```python
from build123d import *

# Parameters (mm, degrees)
SKETCH1_R           = 0.46989906
SKETCH1_R_2         = 0.2499995
BOSS_EXTRUDE1_DEPTH = 1.6764


with BuildPart() as part:
    # Sketch1 → Boss-Extrude1 (new body)
    with BuildSketch(Plane(origin=(0, 0, 0), x_dir=(1, 0, 0), z_dir=(0, 1, 0))):
        with BuildLine():
            Line((73.134188992, 51.586783601), (72.472390316, 51.586783601))
            ThreePointArc((72.472390316, 51.586783601), (72.466796066, 51.573277888), (72.453290354, 51.567683639))
            ThreePointArc((72.453290354, 51.567683639), (72.439692672, 51.573370488), (72.434192176, 51.587044615))
            ThreePointArc((72.434192176, 51.587044615), (71.958321344, 51.791813191), (71.753552768, 52.267684022))
            ThreePointArc((71.753552768, 52.267684022), (71.739878641, 52.273184519), (71.734191792, 52.286782201))
            ThreePointArc((71.734191792, 52.286782201), (71.739786041, 52.300287913), (71.753291754, 52.305882163))
            Line((71.753291754, 52.305882163), (71.753291754, 53.067680639))
            ThreePointArc((71.753291754, 53.067680639), (71.739786041, 53.073274888), (71.734191792, 53.086780601))
            ThreePointArc((71.734191792, 53.086780601), (71.73975368, 53.100253874), (71.753200111, 53.105880343))
            ThreePointArc((71.753200111, 53.105880343), (71.167492925, 54.500977772), (69.772395496, 55.086684958))
            ThreePointArc((69.772395496, 55.086684958), (69.766769027, 55.073238527), (69.753295754, 55.067676639))
            ThreePointArc((69.753295754, 55.067676639), (69.739790041, 55.073270888), (69.734195792, 55.086776601))
            Line((69.734195792, 55.086776601), (57.253320754, 55.086776601))
            ThreePointArc((57.253320754, 55.086776601), (55.845892561, 54.507714506), (55.253416396, 53.105880343))
            ThreePointArc((55.253416396, 53.105880343), (55.266862828, 53.100253874), (55.272424716, 53.086780601))
            ThreePointArc((55.272424716, 53.086780601), (55.266830466, 53.073274888), (55.253324754, 53.067680639))
            Line((55.253324754, 53.067680639), (55.253324754, 41.105904563))
            ThreePointArc((55.253324754, 41.105904563), (55.266830466, 41.100310313), (55.272424716, 41.086804601))
            ThreePointArc((55.272424716, 41.086804601), (55.266862828, 41.073331328), (55.253416396, 41.067704859))
            ThreePointArc((55.253416396, 41.067704859), (55.845892561, 39.665870695), (57.253320754, 39.086808601))
            Line((57.253320754, 39.086808601), (69.734195792, 39.086808601))
            ThreePointArc((69.734195792, 39.086808601), (69.739790041, 39.100314313), (69.753295754, 39.105908563))
            ThreePointArc((69.753295754, 39.105908563), (69.766769027, 39.100346675), (69.772395496, 39.086900243))
            ThreePointArc((69.772395496, 39.086900243), (71.167492925, 39.672607429), (71.753200111, 41.067704859))
            ThreePointArc((71.753200111, 41.067704859), (71.73975368, 41.073331328), (71.734191792, 41.086804601))
            ThreePointArc((71.734191792, 41.086804601), (71.739786041, 41.100310313), (71.753291754, 41.105904563))
            Line((71.753291754, 41.105904563), (71.753291754, 41.867703039))
            ThreePointArc((71.753291754, 41.867703039), (71.739786041, 41.873297288), (71.734191792, 41.886803001))
            ThreePointArc((71.734191792, 41.886803001), (71.739878641, 41.900400683), (71.753552768, 41.905901179))
            ThreePointArc((71.753552768, 41.905901179), (71.958321344, 42.381772011), (72.434192176, 42.586540587))
            ThreePointArc((72.434192176, 42.586540587), (72.439692672, 42.600214713), (72.453290354, 42.605901563))
            ThreePointArc((72.453290354, 42.605901563), (72.466796066, 42.600307313), (72.472390316, 42.586801601))
            Line((72.472390316, 42.586801601), (73.134188992, 42.586801601))
            ThreePointArc((73.134188992, 42.586801601), (73.139783241, 42.600307313), (73.153288954, 42.605901563))
            ThreePointArc((73.153288954, 42.605901563), (73.166754144, 42.600347714), (73.172388573, 42.586916043))
            ThreePointArc((73.172388573, 42.586916043), (74.284646691, 43.055440663), (74.753171311, 44.167698782))
            ThreePointArc((74.753171311, 44.167698782), (74.73973964, 44.173333211), (74.734185792, 44.186798401))
            ThreePointArc((74.734185792, 44.186798401), (74.739780041, 44.200304113), (74.753285754, 44.205898363))
            Line((74.753285754, 44.205898363), (74.753285754, 49.967686839))
            ThreePointArc((74.753285754, 49.967686839), (74.739780041, 49.973281088), (74.734185792, 49.986786801))
            ThreePointArc((74.734185792, 49.986786801), (74.73973964, 50.000251991), (74.753171311, 50.00588642))
            ThreePointArc((74.753171311, 50.00588642), (74.284646691, 51.118144538), (73.172388573, 51.586669158))
            ThreePointArc((73.172388573, 51.586669158), (73.166754144, 51.573237487), (73.153288954, 51.567683639))
            ThreePointArc((73.153288954, 51.567683639), (73.139783241, 51.573277888), (73.134188992, 51.586783601))
        make_face()
        with Locations((57.253320754, 40.586805601)):
            Circle(SKETCH1_R, mode=Mode.SUBTRACT)
        with Locations((69.653295954, 40.786805201)):
            Circle(SKETCH1_R, mode=Mode.SUBTRACT)
        with Locations((69.553296154, 44.486797801)):
            Circle(SKETCH1_R_2, mode=Mode.SUBTRACT)
        with Locations((69.553296154, 45.756795261)):
            Circle(SKETCH1_R_2, mode=Mode.SUBTRACT)
        with Locations((69.553296154, 47.026792721)):
            Circle(SKETCH1_R_2, mode=Mode.SUBTRACT)
        with Locations((58.153318954, 51.986782801)):
            Circle(SKETCH1_R, mode=Mode.SUBTRACT)
        with Locations((69.553296154, 48.296790181)):
            Circle(SKETCH1_R_2, mode=Mode.SUBTRACT)
        with Locations((69.553296154, 49.566787641)):
            Circle(SKETCH1_R_2, mode=Mode.SUBTRACT)
        with Locations((69.553296154, 50.836785101)):
            Circle(SKETCH1_R_2, mode=Mode.SUBTRACT)
        with Locations((69.753295754, 53.586779601)):
            Circle(SKETCH1_R, mode=Mode.SUBTRACT)
    extrude(amount=BOSS_EXTRUDE1_DEPTH)


solid = part.part
```
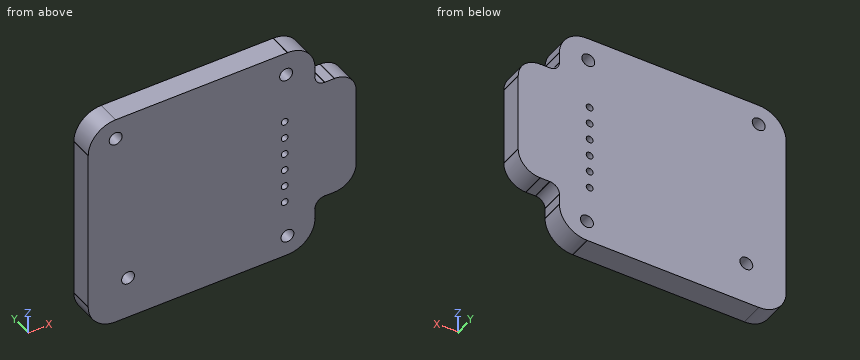
The listing builds one solid part. Answer for the finished solid, in the listing's coordinates (mm). Coordinates: 2 decimals unless noted, no trailing zeros. Loops run counter-clockwise (first coordinate to the right, second up) from the corner with the lowest first, then second, coordinate; pieces in that order, holes last. Notation, with made-up numbers: M 57.25,-3 L 63.25,-3 A38 cw 63.25,36 Z; hole C -31.75,40 d7. An arc over 180 degrees is marked long. Answer as a JSON object with one key per item and string values. Group by question number.
Item 1: Section A-A (z = -41.5) is taken. Write down the section's boundary in (x, y).
Item 2: Section C-C (x = 71) is taken. Write down the section's boundary in (y, z).
Item 3: Consider L1, parallel to X at y = 0.75, z = -44.5; L2, parallel to X at y = 0.1, z = -52; L3, parallel to Z at x = 57.5, y = 1.55. Determine where each line is inside the solid, lowest interval first.
Item 4: This flat-tipped pin is pushed along its axis until it touches: P1, Ø0.5, axis at x = 73, y = 1, coming from the -Z side. Where does it stop, or does it pass through?
Item 5: Section B-B (y = 1.35) is taken. Give the number of separate pieces and of enclosed holes in the cut face, and give its area (3 significant figures).
Solved:
{
 "1": {"outline": "M 55.25,0 L 71.75,0 L 71.75,1.68 L 55.25,1.68 Z"},
 "2": {"outline": "M 0,-54.65 L 1.68,-54.65 L 1.68,-39.52 L 0,-39.52 Z"},
 "3": {"L1": "x = 55.25 to 69.3, 69.8 to 74.75", "L2": "x = 55.25 to 57.68, 58.62 to 71.81", "L3": "z = -55.09 to -40.99, -40.19 to -39.09"},
 "4": {"P1": "stops at z = -51.59"},
 "5": {"separate pieces": "1", "enclosed holes": "10", "area": "283 mm2"}
}
